Input: part model. Units: mm. Frame: model coordinates. Face numbers are marked on the shaded views. A direction names the side the tool comes from. Coordinates: 2 decimals unless noted, no trailing zeros. Loops run counter-clockwise (first coordinate to the right, second up) from the corner with the lowest first, then second, coordinate; pieces in that order, holes last. Notation, with made-up numbers: M -12.75,85 L -0.75,85 A27 cw -0.75,123 Z; hole C -2,65 d9. An arc over 180 degrees is marked long. Use a Markdown table: item, result. Add a question column.
1. Set-up query: the marked faces 1 and 2. Return all of +Z, -Z, +X, -X, +Y, -Y with unobstructed straight access to the full face (end or side cutting, diameter ignored); none if empty.
2. Pin query (flat end, axial travel): pin 1 (1 mm diameter, centred on y = -3, z = 4.5, fed in from -X); pin 2 (0.9 mm diameter, centred on y = 0.5, z = 3, fed in from -X); pin 3 (1.5 mm diameter, centred on y = 0, z = 3, fed in from +X). Return the tip coordinate at first contact, or that it passes through.
3. Section D-D on x = -2.5. Output: boundary loops of the cut face in (y, z).
4. Section C-C on x = 0. Output: boundary loops of the cut face in (y, z).
5. Section A-A on z = 4.1. Output: boundary loops of the cut face in (x, y).
6. Draft query along X for the marked faces 3, 4, 5 and 6. Return one class per face: +X half, -X half, draft (parallel to the pull), parting line (faces both ways), or undercut.
7. Section B-B on y = 0. Output: boundary loops of the cut face in (x, z), then the cut area to 4 significant figures.
8. Line query: L1, parallel to Z at x = -2.75, y = 3.5; L2, parallel to X at y = 2, z = 3.4; L3, parallel to Z at x = 2.75, y = -2. Output: solid intervals per line, ascending. Write a range as [from, to].
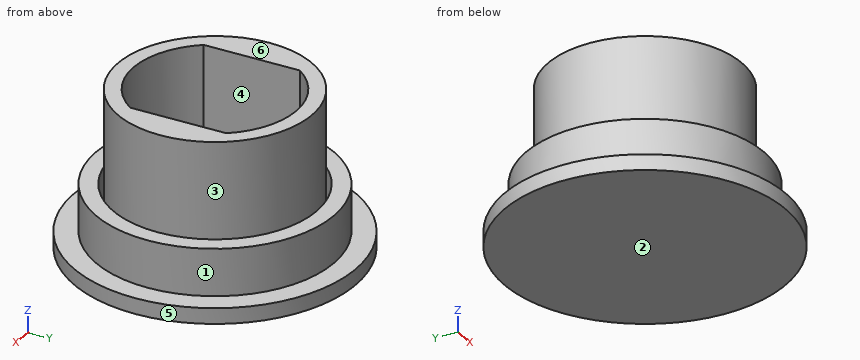
```python
from build123d import *

# Parameters (mm, degrees)
F0_R     = 4.5
F0_R_2   = 3.8
F0_R_3   = 3.25
F1_DEPTH = 0.5
F2_DEPTH = 2
F3_R     = 3.1
F4_DEPTH = 5
F5_DEPTH = 0.5


with BuildPart() as f1:
    # F0 (on Top) → F1 (new body)
    with BuildSketch(Plane.XY):
        Circle(F0_R)
        Circle(F0_R_2, mode=Mode.SUBTRACT)
        Circle(F0_R_2)
        Circle(F0_R_3, mode=Mode.SUBTRACT)
    extrude(amount=F1_DEPTH)

    # F0 (on Top) → F2 (join)
    with BuildSketch(Plane.XY):
        Circle(F0_R_2)
        Circle(F0_R_3, mode=Mode.SUBTRACT)
    extrude(amount=F2_DEPTH)



with BuildPart() as f4:
    # F3 (on face) → F4 (new body)
    with BuildSketch(Plane.XY):
        Circle(F3_R)
        with BuildLine():
            ThreePointArc((2.1, 1.5329709717), (2.4718414189, 0.8062257748), (2.6, 0))
            ThreePointArc((2.6, 0), (2.4718414189, -0.8062257748), (2.1, -1.5329709717))
            ThreePointArc((2.1, -1.5329709717), (0, -2.6), (-2.1, -1.5329709717))
            ThreePointArc((-2.1, -1.5329709717), (-2.6, 0), (-2.1, 1.5329709717))
            ThreePointArc((-2.1, 1.5329709717), (0, 2.6), (2.1, 1.5329709717))
        make_face(mode=Mode.SUBTRACT)
        with BuildLine():
            ThreePointArc((2.1, -1.5329709717), (2.4718414189, -0.8062257748), (2.6, 0))
            ThreePointArc((2.6, 0), (2.4718414189, 0.8062257748), (2.1, 1.5329709717))
            Line((2.1, 1.5329709717), (2.1, -1.5329709717))
        make_face()
        with BuildLine():
            Line((-2.1, -1.5329709717), (-2.1, 1.5329709717))
            ThreePointArc((-2.1, 1.5329709717), (-2.6, 0), (-2.1, -1.5329709717))
        make_face()
    extrude(amount=F4_DEPTH)


with BuildPart() as f1_1:
    add(f1.part)

    add(f4.part)  # F5 merges F4
    # F0 (on Top) → F5 (join)
    with BuildSketch(Plane.XY):
        Circle(F0_R_3)
    extrude(amount=F5_DEPTH)


solid = f1_1.part
```
Answers below:
| question | item | result |
|---|---|---|
| 1 | face 1 | +Z |
| 1 | face 2 | -Z, +X, -X, +Y, -Y |
| 2 | pin 1 | stops at x = -1.83 |
| 2 | pin 2 | stops at x = -3.1 |
| 2 | pin 3 | stops at x = 3.1 |
| 3 | outline | M -3.74,0 L 3.74,0 L 3.74,0.5 L 2.86,0.5 L 2.86,2 L 2.08,2 L 2.08,0.5 L 1.83,0.5 L 1.83,5 L -1.83,5 L -1.83,0.5 L -2.08,0.5 L -2.08,2 L -2.86,2 L -2.86,0.5 L -3.74,0.5 Z |
| 4 | outline | M -4.5,0 L 4.5,0 L 4.5,0.5 L 3.8,0.5 L 3.8,2 L 3.25,2 L 3.25,0.5 L 3.1,0.5 L 3.1,5 L 2.6,5 L 2.6,0.5 L -2.6,0.5 L -2.6,5 L -3.1,5 L -3.1,0.5 L -3.25,0.5 L -3.25,2 L -3.8,2 L -3.8,0.5 L -4.5,0.5 Z |
| 5 | outline | C 0,0 d6.2; hole M -2.1,-1.53 A2.6 ccw 2.1,-1.53 L 2.1,1.53 A2.6 ccw -2.1,1.53 Z |
| 6 | face 3 | undercut |
| 6 | face 4 | undercut |
| 6 | face 5 | parting line |
| 6 | face 6 | draft |
| 7 | outline | M -4.5,0 L 4.5,0 L 4.5,0.5 L 3.8,0.5 L 3.8,2 L 3.25,2 L 3.25,0.5 L 3.1,0.5 L 3.1,5 L 2.1,5 L 2.1,0.5 L -2.1,0.5 L -2.1,5 L -3.1,5 L -3.1,0.5 L -3.25,0.5 L -3.25,2 L -3.8,2 L -3.8,0.5 L -4.5,0.5 Z |
| 7 | area | 15.15 mm² |
| 8 | L1 | z = [0, 0.5] |
| 8 | L2 | x = [-2.37, -1.66], [1.66, 2.37] |
| 8 | L3 | z = [0, 2] |
